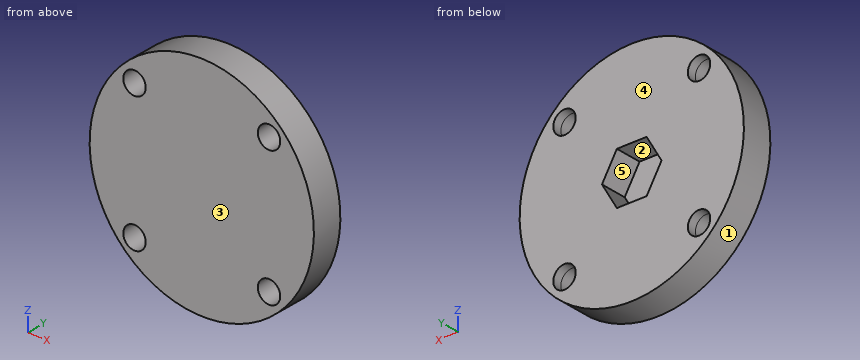
```python
from build123d import *

# Parameters (mm, degrees)
SKETCH1_R           = 25
BOSS_EXTRUDE1_DEPTH = 5
SKETCH2_R           = 2.5
CUT_EXTRUDE1_DEPTH  = 36.707142143
CUT_EXTRUDE2_DEPTH  = 4
MOVE_FACE1_BY       = 2
MOVE_START          = 1
MOVE_FACE2_DEPTH    = 6


# Read off the part's stored shape, not the designer's step: Move Face2
with BuildPart() as part:
    # Sketch1 → Boss-Extrude1 (new body)
    with BuildSketch(Plane(origin=(0, 0, 0), x_dir=(1, 0, 0), z_dir=(0, 1, 0))):
        with Locations(Location((0, 0, 0), (0, 0, 270))):
            Circle(SKETCH1_R)
    extrude(amount=BOSS_EXTRUDE1_DEPTH)

    # Sketch2 → Cut-Extrude1 (cut, through all)
    with BuildSketch(Plane(origin=(0, 5, 0), x_dir=(1, 0, 0), z_dir=(0, 1, 0))):
        with Locations(Location((-15, 15, 0), (0, 0, 270))):
            Circle(SKETCH2_R)
        with Locations(Location((15, 15, 0), (0, 0, 270))):
            Circle(SKETCH2_R)
        with Locations(Location((15, -15, 0), (0, 0, 270))):
            Circle(SKETCH2_R)
        with Locations(Location((-15, -15, 0), (0, 0, 270))):
            Circle(SKETCH2_R)
    extrude(amount=-CUT_EXTRUDE1_DEPTH, mode=Mode.SUBTRACT)

    # Sketch7 → Cut-Extrude2 (cut)
    with BuildSketch(Plane(origin=(0, 5, 0), x_dir=(1, 0, 0), z_dir=(0, 1, 0))):
        Polygon((3.262029021, -5.65), (-3.262029021, -5.65), (-6.524058042, 0), (-3.262029021, 5.65), (3.262029021, 5.65), (6.524058042, 0), align=None)
    extrude(amount=-CUT_EXTRUDE2_DEPTH, mode=Mode.SUBTRACT)

    # Move Face1: a face moved outward by 2.0
    extrude(part.faces().sort_by_distance((0, 5, 12.5))[0], amount=MOVE_FACE1_BY, dir=(0, 1, 0))

    # Move Face2 outline → Move Face2 (cut)
    with BuildSketch(Plane(origin=(0, 0, 0), x_dir=(1, 0, 0), z_dir=(0, 1, 0)).offset(MOVE_START)):
        Polygon((-3.319764048, 5.75), (-6.639528096, 0), (-3.319764048, -5.75), (3.319764048, -5.75), (6.639528096, 0), (3.319764048, 5.75), align=None)
        Polygon((-3.262029021, -5.65), (-6.524058042, 0), (-3.262029021, 5.65), (3.262029021, 5.65), (6.524058042, 0), (3.262029021, -5.65), align=None, mode=Mode.SUBTRACT)
    extrude(amount=MOVE_FACE2_DEPTH, mode=Mode.SUBTRACT)


solid = part.part
```
Source: CAD feature listing. Evaluate the final solid. Frame: model axes, mm. Face numbers are marked on the shaded views. A direction names the side the tool comes from. Coordinates: 2 decimals unless noted, no trailing zeros. Loops run counter-clockwise (first coordinate to the right, second up) from the corner with the lowest first, then second, coordinate; pieces in that order, holes last. Notation, with made-up numbers: (23, -28) -> (80, -28) arc R25 cw to (80, -6) -> close; hole circle Ø8 at (80, 32.5). An arc over 180 degrees is marked (long way). One line per item, written item: value. Start each with the question number.
Q1. Section query C-C, the plane z = -15. Return the cut outline in (x, y), and give its area (3 significant figures).
Q2. Section query A-A, the plane y = 3. Return the cut outline in (x, z), and give its area (3 significant figures).
Q3. Line query: line 1 along X through (y, z) = (1.6, -15); line 2 along X through (y, z) = (6.25, 13); line 3 along Z through (x, y) = (-0.5, 2.75) (3 decimals). Output: solid intervals per line, ascending.
Q4. Contact query for flat-ended pins moving along their axis: P1, Ø4, axis at x = -15, z = -15, coming from the -Y side; P2, Ø4, axis at x = 19, y = 4, coming from the -Z side; P3, Ø3, axis at x = -14, y = 1.5, coming from the +Z side. Output: stop coordinate, or through.
Q5. Set-up query: the marked faces 4 and 5. Return all of +Z, -Z, +X, -X, +Y, -Y with unobstructed straight access to the full face (end or side cutting, diameter ignored); none if empty.
Q6. Section query B-B, the plane x = -15. Return the cut outline in (y, z).
Q7. Mould query, pull axis X, two halves, no side actions, for the marked faces 1, 2 and 3. Classes: pulls with the +X half, pulls with the -X half, needs draft (parallel to the pull), parting line crosses it, or undercut.
Q8. Section query D-D, the plane x = 4.5. Return the cut outline in (y, z), and give its area (3 significant figures).
Results:
1. outline: (-20, 0) -> (-17.5, 0) -> (-17.5, 7) -> (-20, 7) -> close; (-12.5, 0) -> (12.5, 0) -> (12.5, 7) -> (-12.5, 7) -> close; (17.5, 0) -> (20, 0) -> (20, 7) -> (17.5, 7) -> close
1. area: 210 mm^2
2. outline: circle Ø50 at (0, 0); hole circle Ø5 at (-15, -15); hole circle Ø5 at (-15, 15); hole (-6.64, 0) -> (-3.32, -5.75) -> (3.32, -5.75) -> (6.64, 0) -> (3.32, 5.75) -> (-3.32, 5.75) -> close; hole circle Ø5 at (15, -15); hole circle Ø5 at (15, 15)
2. area: 1,770 mm^2
3. line 1: -20 to -17.5, -12.5 to 12.5, 17.5 to 20
3. line 2: -21.35 to -16.5, -13.5 to 13.5, 16.5 to 21.35
3. line 3: -24.995 to -5.75, 5.75 to 24.995
4. P1: through
4. P2: z = -18.33
4. P3: z = 21.65
5. face 4: +Z, -Z, +X, -X, +Y
5. face 5: +Y
6. outline: (0, -20) -> (7, -20) -> (7, -17.5) -> (0, -17.5) -> close; (0, -12.5) -> (7, -12.5) -> (7, 12.5) -> (0, 12.5) -> close; (0, 17.5) -> (7, 17.5) -> (7, 20) -> (0, 20) -> close
7. face 1: parting line crosses it
7. face 2: undercut
7. face 3: needs draft
8. outline: (0, -24.59) -> (7, -24.59) -> (7, -3.71) -> (1, -3.71) -> (1, 3.71) -> (7, 3.71) -> (7, 24.59) -> (0, 24.59) -> close
8. area: 300 mm^2
